Can you work these out from the model? Positions are in its coordinate system, mm. Face numbers are marked on the shaded views. Round coordinates to 2 decimals unless told otherwise and drop trailing zeros. Loops run counter-clockwise (first coordinate to the right, second up) from the corner with the lowest first, then second, coordinate; pieces in that order, holes last. Notation, with made-up numbers: (29.5, -18) -> (72.5, -18) arc R11 ccw to (72.5, 2) -> close; hole circle Ø4 at (-22, 84). An arc over 180 degrees is marked (long way). Write each question's results on one line, items separated by ' | '.
from build123d import *

# Parameters (mm, degrees)
SKETCH004_W   = 1905
SKETCH004_H   = 800
PAD001_DEPTH  = 18
SKETCH006_W   = 1905
SKETCH006_H   = 100
SKETCH006_W_2 = 90
SKETCH006_H_2 = 400
PAD002_DEPTH  = 18
SKETCH005_R   = 28
POCKET_DEPTH  = 40
FILLET002_R   = 9.2
CHAMFER_SIZE  = 20
FILLET003_R   = 9.2


with BuildPart() as part:
    # Sketch004 → Pad001 (new body)
    with BuildSketch(Plane.XY):
        Rectangle(SKETCH004_W, SKETCH004_H)
    extrude(amount=PAD001_DEPTH)

    # Sketch006 (on Face5 of Pad001) → Pad002 (join)
    with BuildSketch(Plane(origin=(0, 0, 0), x_dir=(1, 0, 0), z_dir=(0, 0, -1))):
        with Locations((0, 350)):
            Rectangle(SKETCH006_W, SKETCH006_H)
        Polygon((952.5, -300), (952.5, -400), (-952.5, -400), (-952.5, -300), (-747.5, -300), (-747.5, -250), (-657.5, -250), (-657.5, -300), (657.5, -300), (657.5, -250), (747.5, -250), (747.5, -300), align=None)
        with Locations((-907.5, 30)):
            Rectangle(SKETCH006_W_2, SKETCH006_H_2)
        with Locations((907.5, 30)):
            Rectangle(SKETCH006_W_2, SKETCH006_H_2)
    extrude(amount=PAD002_DEPTH)

    # Sketch005 (on Face6 of Pad001) → Pocket (cut)
    with BuildSketch(Plane.XY.offset(18)):
        with Locations((-702.5, 300)):
            Circle(SKETCH005_R)
        with Locations((702.5, 300)):
            Circle(SKETCH005_R)
    extrude(amount=-POCKET_DEPTH, mode=Mode.SUBTRACT)

    # Fillet002
    fillet002_edges = [part.edges().sort_by_distance(p)[0] for p in [
        (674.5, 300, -18),
        (-730.5, 300, -18),
        (-730.5, 300, 18),
        (674.5, 300, 18),
    ]]
    fillet(fillet002_edges, radius=FILLET002_R)

    # Chamfer
    chamfer_edges = [part.edges().sort_by_distance(p)[0] for p in [
        (0, -400, 18),
    ]]
    chamfer(chamfer_edges, length=CHAMFER_SIZE)

    # Fillet003
    fillet003_edges = [part.edges().sort_by_distance(p)[0] for p in [
        (0, -400, -18),
        (0, -400, -2),
        (0, -380, 18),
    ]]
    fillet(fillet003_edges, radius=FILLET003_R)


solid = part.part
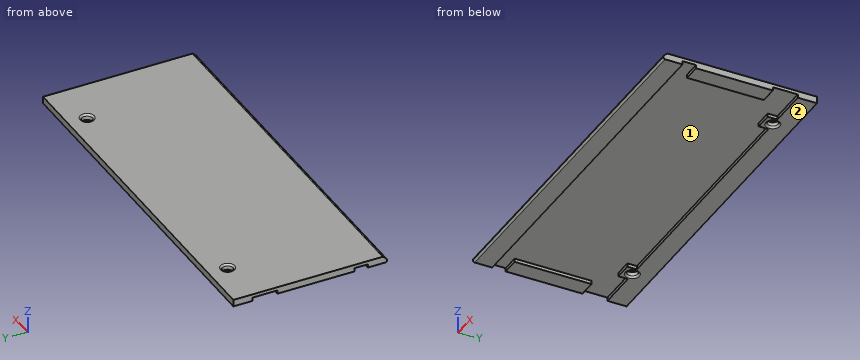
1. We'd pull the mould along Y, two halves only. Please class the marked faces 1 and 2: pulls with the +Y half, pulls with the -Y half, needs draft (parallel to the pull), parting line crosses it, or undercut.
Final values:
face 1: undercut | face 2: needs draft
2. If we section it at C-C (x = -189.5): List the corners of the cut face in (y, z) for me, then the cut area to 3 significant figures.
Final values:
outline: (-400, -8.8) arc R9.2 ccw to (-390.8, -18) -> (-300, -18) -> (-300, 0) -> (300, 0) -> (300, -18) -> (400, -18) -> (400, 18) -> (-376.19, 18) arc R9.2 ccw to (-382.69, 15.31) -> (-397.31, 0.69) arc R9.2 ccw to (-400, -5.81) -> close | area: 17,800 mm2
3. Please list where these lines run through material, in increasing order: line 1 (X direction, y = -14, z = -5.5); line 2 (Y direction, x = 866.5, z = -6); line 3 (Y direction, x = -702.5, z = -2.25). Write a range as from..to.
Final values:
line 1: -952.5..-862.5, 862.5..952.5 | line 2: -400..-300, -230..170, 300..400 | line 3: -399.28..-300, 250..272, 328..400
4. If we section it at B-B (y = -176.5): List the corners of the cut face in (x, z) for me.
Final values:
outline: (-952.5, -18) -> (-862.5, -18) -> (-862.5, 0) -> (862.5, 0) -> (862.5, -18) -> (952.5, -18) -> (952.5, 18) -> (-952.5, 18) -> close
5. If we section it at A-A (x = 702.5): List the corners of the cut face in (y, z) for me.
Final values:
outline: (-400, -8.8) arc R9.2 ccw to (-390.8, -18) -> (-300, -18) -> (-300, 0) -> (250, 0) -> (250, -18) -> (262.8, -18) arc R9.2 ccw to (272, -8.8) -> (272, 8.8) arc R9.2 ccw to (262.8, 18) -> (-376.19, 18) arc R9.2 ccw to (-382.69, 15.31) -> (-397.31, 0.69) arc R9.2 ccw to (-400, -5.81) -> close; (328, -8.8) arc R9.2 ccw to (337.2, -18) -> (400, -18) -> (400, 18) -> (337.2, 18) arc R9.2 ccw to (328, 8.8) -> close
6. Will this pin go through, and if not, where does the flat tip stop? pin 1 (1.5 mm diameter, centred on x = 657.5, z = 3, fed in from -Y).
Final values:
pin 1: y = -395.75
7. If we section it at D-D (y = -279): List the corners of the cut face in (x, z) for me.
Final values:
outline: (-952.5, 0) -> (952.5, 0) -> (952.5, 18) -> (-952.5, 18) -> close
